Autodesk Inventor part; units mm, degrees
ref_plane "Work Plane1" through (-104.8982, -25.3956, -49) normal (0, 0, 1) x (1, 0, 0)
ref_plane "YZ Plane" through (0, 0, 0) normal (1, 0, 0) x (0, 1, 0)
ref_plane "XZ Plane" through (0, 0, 0) normal (0, 1, 0) x (-1, 0, 0)
sketch "Sketch1" plane through (0, 0, 0) normal (0, 0, 1) x (1, 0, 0)
  arc A0 (68.5, 19.5) -> (65.5, 22.5) centre (65.5, 19.5) ccw
  line L0 (-65.5, 22.5) -> (65.5, 22.5)
  arc A1 (-65.5, 22.5) -> (-68.5, 19.5) centre (-65.5, 19.5) ccw
  line L1 (-68.5, -19.5) -> (-68.5, 19.5)
  arc A2 (-68.5, -19.5) -> (-65.5, -22.5) centre (-65.5, -19.5) ccw
  line L2 (65.5, -22.5) -> (-65.5, -22.5)
  arc A3 (65.5, -22.5) -> (68.5, -19.5) centre (65.5, -19.5) ccw
  line L3 (68.5, 19.5) -> (68.5, -19.5)
  line L4 (88.6498, -25.3956) -> (-89.1502, -25.3956)
  line L5 (-89.1502, -25.3956) -> (-89.1502, 25.4044)
  line L6 (-89.1502, 25.4044) -> (88.6498, 25.4044)
  line L7 (88.6498, 25.4044) -> (88.6498, -25.3956)
  line L8 (-0.2502, 266.6127) -> (-0.2502, -243.9407)
  point P0 (0, 0)
  dimension "d23" = 177.8
  dimension "d24" = 50.8
ref_plane "Work Plane1" through (-104.8982, -25.3956, -49) normal (0, 0, 1) x (1, 0, 0)
extrude "Extrusion1" add sketch "Sketch1" against normal up to surface (49 mm away) contours A0 L0 L8 L6 L7 L4 L2 A3 L3 | L0 A1 L1 A2 L2 L8 L4 L5 L6
sketch "Sketch2" plane through (0, 0, 0) normal (0, 0, 1) x (1, 0, 0)
  line L0 (88.6498, -25.3956) -> (88.6498, 25.4044)
  line L1 (-89.1502, 25.4044) -> (-89.1502, -25.3956)
  arc A0 (68.5, 19.5) -> (65.5, 22.5) centre (65.5, 19.5) ccw
  line L2 (68.5, 19.5) -> (68.5, -19.5)
  arc A1 (65.5, -22.5) -> (68.5, -19.5) centre (65.5, -19.5) ccw
  line L3 (65.5, -22.5) -> (-65.5, -22.5)
  arc A2 (-68.5, -19.5) -> (-65.5, -22.5) centre (-65.5, -19.5) ccw
  line L4 (-68.5, -19.5) -> (-68.5, 19.5)
  arc A3 (-65.5, 22.5) -> (-68.5, 19.5) centre (-65.5, 19.5) ccw
  line L5 (-65.5, 22.5) -> (65.5, 22.5)
  line L6 (65.5, 22.5) -> (-65.5, 22.5)
  line L7 (-65.5, 22.5) -> (-73.2752, 22.5)
  line L8 (-73.2752, 22.5) -> (-73.2752, 8.8856)
  line L9 (-73.2752, 8.8856) -> (-81.5302, 8.8856)
  line L10 (-81.5302, 8.8856) -> (-81.5302, -8.8944)
  line L11 (-81.5302, -8.8944) -> (-73.2752, -8.8944)
  line L12 (-73.2752, -8.8944) -> (-73.2752, -22.5088)
  line L13 (-73.2752, -22.5088) -> (72.7748, -22.5088)
  line L14 (72.7748, -22.5088) -> (72.7748, -8.8944)
  line L15 (72.7748, -8.8944) -> (81.0298, -8.8944)
  line L16 (81.0298, -8.8944) -> (81.0298, 8.8856)
  line L17 (81.0298, 8.8856) -> (72.7748, 8.8856)
  line L18 (72.7748, 8.8856) -> (72.7748, 22.5)
  line L19 (-65.5, 22.5) -> (72.7748, 22.5)
  line L20 (88.6498, 25.4044) -> (-89.1502, 25.4044)
  line L21 (-89.1502, -25.3956) -> (88.6498, -25.3956)
  point P0 (0, 0)
  dimension "d4" = 45.0088
  dimension "d5" = 17.78
  dimension "d6" = 7.62
  dimension "d7" = 7.62
  dimension "d8" = 146.05
extrude "Extrusion2" cut sketch "Sketch2" against normal up to next contours A0 L19 L18 L17 L16 L15 L14 L13 L12 L11 L10 L9 L8 L7 A3 L4 A2 L3 A1 L2
sketch "Sketch5" plane through (88.6498, 25.4044, -49) normal (0, 0, -1) x (-1, 0, 0)
  line L0 (0, 0) -> (0, -50.8)
  line L1 (177.8, -50.8) -> (0, -50.8)
  line L2 (0, 0) -> (177.8, 0)
  line L3 (177.8, 0) -> (177.8, -50.8)
  line L4 (177.8, -50.8) -> (0, -50.8)
  line L5 (0, -50.8) -> (0, 0)
  point P0 (88.6498, -25.4044)
fillet "Fillet2" radius 3.175 12 edges at (-73.2752, 8.8856, -24.5) (-73.2752, 22.5, -24.5) (-81.5302, 8.8856, -24.5) (-81.5302, -8.8944, -24.5) (-73.2752, -8.8944, -24.5) (-73.2752, -22.5088, -24.5) (72.7748, -22.5088, -24.5) (72.7748, -8.8944, -24.5) (81.0298, -8.8944, -24.5) (81.0298, 8.8856, -24.5) (72.7748, 8.8856, -24.5) (72.7748, 22.5, -24.5)
sketch "Sketch6" plane through (0, 0, 0) normal (0, 0, 1) x (1, 0, 0)
  line L0 (-89.1502, 25.4044) -> (-89.1502, -25.3956)
  line L1 (-89.1502, -25.3956) -> (88.6498, -25.3956)
  line L2 (88.6498, 25.4044) -> (-89.1502, 25.4044)
  line L3 (88.6498, -25.3956) -> (88.6498, 25.4044)
  point P0 (0, 0)
  point P1 (-81.2127, 17.1494)
  point P2 (-81.2127, -17.1406)
  point P3 (80.6996, -17.1406)
  point P4 (80.6996, 17.1494)
  dimension "d26" = 7.9375
  dimension "d27" = 8.255
  dimension "d28" = 8.255
  dimension "d29" = 7.9502
extrude "Extrusion3" add sketch "Sketch5" along normal blind 1.5875
hole "Hole2" at (-81.2127, 17.1494, 0) at (-81.2127, -17.1406, 0) at (80.6996, -17.1406, 0) at (80.6996, 17.1494, 0) direction (0, 0, -1) diameter 6.35 end through all
fillet "Fillet3" radius 3.175 4 edges at (-89.1502, 25.4044, -25.2938) (-89.1502, -25.3956, -25.2938) (88.6498, 25.4044, -25.2938) (88.6498, -25.3956, -25.2938)
properties part number "Battery Holder" material "PC/ABS Plastic"
CAD build for the part. Positions are in the model's coordinates, mm. A direction names the side the tool comes from. Round coordinates to 2 decimals unless told otherwise and drop trailing zeros. Loops run counter-clockwise (first coordinate to the right, second up) from the corner with the lowest first, then second, coordinate; pieces in that order, holes last. Notation, with made-up numbers: M -10.75,83.5 L 37.25,83.5 A24 cw 37.25,103.5 Z; hole C 82,-17.5 d3. An arc over 180 degrees is marked long. Use a Markdown table: item, result. Add a question column.
(1) Pull direction X, two halves, no side cores. Call faces 1 (the face through (1, 25.404, -25)), 2 (the face through (-89.15, 0, -25)), 3 (the face through (80.124, -7.94, -24.843)): +X half, -X half, draft (parallel to the pull), parting line (faces both ways), or undercut.
(2) Drill centre lines: line 1 (Y direction, x = -56.5, z = -22); line 2 (X direction, y = -19, z = -42); line 3 (X direction, y = -6, z = -1.5). Where is each one in solid material? Low to high.
(3) Cut at C-C (y = 16). Give the cut face in (x, z), and give its area (3 significant figures).
(4) Cut at D-D (z = -39). State how many separate pieces and enclosed holes the cut face has, and give its area (3 significant figures).
(5) Flat gauge pins, fed straight in: pin 1 (3 mm diameter, centred on x = -42, y = 5, fed in from +Z); pin 2 (8.5 mm diameter, centred on x = 80.7, y = -17.14, fed in from -Z). Where does each tip first touch, or does it go through?
(6) Cut at A-A (y = 2). Give the cut face in (x, z).
(7) Which spindle directions (+Z, -Z, +X, -X, +Y, -Y) get a long thin tool onto all of the face, cutting with end or side? Do faces 4 (the face through (-80.575, -7.989, -24.843)), 5 (the face through (-1, 23, 0)). Say none if no direction does.
(8) Cut at B-B (x = 5.5). Give the cut face in (y, z).
Geometry says:
| question | item | result |
|---|---|---|
| 1 | face 1 | draft |
| 1 | face 2 | -X half |
| 1 | face 3 | undercut |
| 2 | line 1 | y = -25.4 to -22.51, 22.5 to 25.4 |
| 2 | line 2 | x = -89.15 to -83.79, -78.64 to -73.28, 72.77 to 78.13, 83.27 to 88.65 |
| 2 | line 3 | x = -89.15 to -81.52, 81.02 to 88.65 |
| 3 | outline | M -89.15,-50.59 L -84.17,-50.59 L -84.17,0 L -89.15,0 Z; M -78.25,-50.59 L 77.74,-50.59 L 77.74,0 L 72.77,0 L 72.77,-49 L -73.28,-49 L -73.28,0 L -78.25,0 Z; M 83.66,-50.59 L 88.65,-50.59 L 88.65,0 L 83.66,0 Z |
| 3 | area | 1,240 mm² |
| 4 | separate pieces | 1 |
| 4 | enclosed holes | 5 |
| 4 | area | 2,040 mm² |
| 5 | pin 1 | stops at z = -49 |
| 5 | pin 2 | stops at z = -50.59 |
| 6 | outline | M -89.15,-50.59 L 88.65,-50.59 L 88.65,0 L 81.03,0 L 81.03,-49 L -81.53,-49 L -81.53,0 L -89.15,0 Z |
| 7 | face 4 | +Z |
| 7 | face 5 | +Z, +X, -X, +Y, -Y |
| 8 | outline | M -25.4,-50.59 L 25.4,-50.59 L 25.4,0 L 22.5,0 L 22.5,-49 L -22.51,-49 L -22.51,0 L -25.4,0 Z |
